The drawing under review shows one solid part. Ordinate dimensions are in mm from its lowest x, y, z. A direction names the side the tool comes from. Round coordinates to 2 decimals unless told otherwise and drop trailing zeros. Loops run counter-clockwise (first coordinate to the right, second up) from the corner with the lowest first, then second, coordinate; pieces in that order, holes last. Notation, with made-up numbers: (46.25, 42.25) - (76.25, 42.25) arc R22 ccw to (76.25, 69.25) - close; hole circle Ø7 at (45.5, 60.5). An arc over 180 degrees is marked (long way). Answer as CSV lines item,"result".
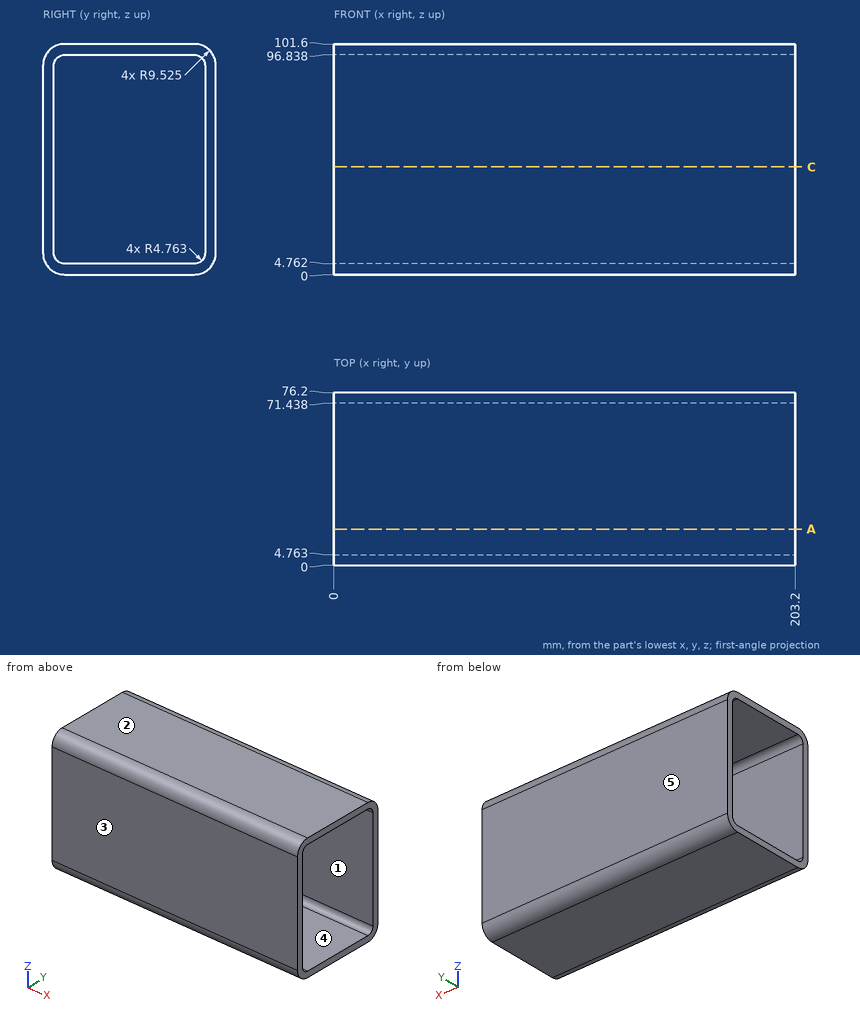
1. Tool access review of the marked faces 4 and 5: name each direction out of +Z, -Z, +X, -X, +Y, -Y from which nothing blocks a thin tool from reaching the whole face with its end or side.
Numbers:
face 4,"+X, -X"
face 5,"+Z, -Z, +X, -X, +Y"
2. Clearance check with flat-ended pins moving along their axes: pin 1 (12 mm diameter, centred on x = 97, y = 20, fed in from -Z); pin 2 (10 mm diameter, centred on y = 33.5, z = 12.5, fed in from +X). State where each tip first meets the part, or that it passes through.
Numbers:
pin 1,"stops at z = 0"
pin 2,"passes through"
3. Take a section at C-C (z = 47.5). State the section outline as (x, y) points.
Numbers:
outline,"(0, 0) - (203.2, 0) - (203.2, 4.76) - (0, 4.76) - close; (0, 71.44) - (203.2, 71.44) - (203.2, 76.2) - (0, 76.2) - close"
4. Take a section at A-A (y = 16). State the section outline as (x, z) points.
Numbers:
outline,"(0, 0) - (203.2, 0) - (203.2, 4.76) - (0, 4.76) - close; (0, 96.84) - (203.2, 96.84) - (203.2, 101.6) - (0, 101.6) - close"
5. Wall thickness on probe 1 along Z at (x, y) = (38, 33.5); probe 2 along Y at (x, z) = (42, 91); probe 3 along Z at (x, y) = (78.5, 70.5) (1 decimal): over which ranges is each line inside the solid? List them lowest first.
Numbers:
probe 1,"z = 0 to 4.76, 96.84 to 101.6"
probe 2,"y = 0 to 4.76, 71.44 to 76.2"
probe 3,"z = 0.8 to 6.7, 94.9 to 100.8"
6. Draft analysis for pull direction Z (two halves, no side actions). For the marked faces 1, 2 and 3, state which applies: +Z half, -Z half, draft (parallel to the pull), parting line (faces both ways), or undercut.
Numbers:
face 1,"undercut"
face 2,"+Z half"
face 3,"draft"
